Work out the finished part from the listing and answer in its coordinate system (mm). A direction names the side the tool comes from. Coordinates: 2 decimals unless noted, no trailing zeros. Write each loop counter-clockwise with the first axis right and the second up, starting at its lowest first coordinate (ties: lowest second). Pieces come first, ordered by that corner, then holes. Notation, with made-up numbers: (84.25, 39.25) - (139.25, 39.25) arc R17 ccw to (139.25, 62.25) - close; hole circle Ø3 at (-35, 2). An arc over 180 degrees is marked (long way). Answer as a JSON object with one key per item and string values. Group by question number.
from build123d import *

# Parameters (mm, degrees)
F1_DEPTH = 7
F2_R     = 5
F3_R     = 0.5
F4_R     = 1.5
F5_DEPTH = 8


with BuildPart() as f1:
    # F0 (on Top) → F1 (new body, symmetric)
    with BuildSketch(Plane.XY):
        with BuildLine():
            ThreePointArc((-5, 0), (0, -5), (5, 0))
            ThreePointArc((5, 0), (3.535534, 3.535534), (0, 5))
            ThreePointArc((0, 5), (-3.535534, 3.535534), (-5, 0))
        make_face()
        with BuildLine():
            ThreePointArc((-2.75, 2.165064), (-1.75, 3.031089), (-0.5, 3.464102))
            ThreePointArc((-0.5, 3.464102), (0, 3.5), (0.5, 3.464102))
            ThreePointArc((0.5, 3.464102), (1.75, 3.031089), (2.75, 2.165064))
            Line((2.75, 2.165064), (1.049038, 1.183013))
            Line((1.049038, 1.183013), (1.549038, 0.316987))
            Line((1.549038, 0.316987), (3.25, 1.299038))
            ThreePointArc((3.25, 1.299038), (3.5, 0), (3.25, -1.299038))
            ThreePointArc((3.25, -1.299038), (3.031089, -1.75), (2.75, -2.165064))
            ThreePointArc((2.75, -2.165064), (1.75, -3.031089), (0.5, -3.464102))
            ThreePointArc((0.5, -3.464102), (0, -3.5), (-0.5, -3.464102))
            ThreePointArc((-0.5, -3.464102), (-1.75, -3.031089), (-2.75, -2.165064))
            ThreePointArc((-2.75, -2.165064), (-3.031089, -1.75), (-3.25, -1.299038))
            ThreePointArc((-3.25, -1.299038), (-3.5, 0), (-3.25, 1.299038))
            ThreePointArc((-3.25, 1.299038), (-3.031089, 1.75), (-2.75, 2.165064))
        make_face(mode=Mode.SUBTRACT)
        with BuildLine():
            Line((-1.049038, 1.183013), (-2.75, 2.165064))
            ThreePointArc((-2.75, 2.165064), (-3.031089, 1.75), (-3.25, 1.299038))
            Line((-3.25, 1.299038), (-1.549038, 0.316987))
            Line((-1.549038, 0.316987), (-1.049038, 1.183013))
        make_face()
        with BuildLine():
            ThreePointArc((0.5, 3.464102), (0, 3.5), (-0.5, 3.464102))
            Line((-0.5, 3.464102), (-0.5, 1.5))
            Line((-0.5, 1.5), (0.5, 1.5))
            Line((0.5, 1.5), (0.5, 3.464102))
        make_face()
        with BuildLine():
            Line((-1.549038, -0.316987), (-3.25, -1.299038))
            ThreePointArc((-3.25, -1.299038), (-3.031089, -1.75), (-2.75, -2.165064))
            Line((-2.75, -2.165064), (-1.049038, -1.183013))
            Line((-1.049038, -1.183013), (-1.549038, -0.316987))
        make_face()
        with BuildLine():
            Line((-0.5, -1.5), (-0.5, -3.464102))
            ThreePointArc((-0.5, -3.464102), (0, -3.5), (0.5, -3.464102))
            Line((0.5, -3.464102), (0.5, -1.5))
            Line((0.5, -1.5), (-0.5, -1.5))
        make_face()
        with BuildLine():
            ThreePointArc((2.75, -2.165064), (3.031089, -1.75), (3.25, -1.299038))
            Line((3.25, -1.299038), (1.549038, -0.316987))
            Line((1.549038, -0.316987), (1.049038, -1.183013))
            Line((1.049038, -1.183013), (2.75, -2.165064))
        make_face()
        with BuildLine():
            ThreePointArc((-5, 0), (-3.535534, 3.535534), (0, 5))
            Line((0, 5), (-13, 5))
            Line((-13, 5), (-13, 0))
            Line((-13, 0), (-5, 0))
        make_face()
    extrude(amount=F1_DEPTH, both=True)

    # F2
    f2_edges = [f1.edges().sort_by_distance(p)[0] for p in [
        (-5, 0, 0),
    ]]
    fillet(f2_edges, radius=F2_R)

    # F3
    f3_edges = [f1.edges().sort_by_distance(p)[0] for p in [
        (-13, 5, 0),
        (-13, 0, 0),
    ]]
    fillet(f3_edges, radius=F3_R)

    # F4 (on face) → F5 (cut)
    with BuildSketch(Plane(origin=(-13, 0, 0), x_dir=(0, -1, 0), z_dir=(-1, 0, 0))):
        with Locations((-2.5, 4)):
            Circle(F4_R)
        with Locations((-2.5, -4)):
            Circle(F4_R)
    extrude(amount=-F5_DEPTH, mode=Mode.SUBTRACT)


solid = f1.part
Q1. Flat-ended cylindrical pins translate along their axes: pin 1 Ø1.6 at (y, z) = (2, -2.5) entering from +X; pin 2 Ø0.6 at (y, z) = (-2.5, -2) entering from -X; pin 3 Ø1.9 at (x, z) = (-10, 2) entering from -Y. Find the tip coordinate at first contact, or state that the pin passes through.
Q2. Section B-B on y = 1.75 is taken. Determine the outline of the cut face in (x, z), plus the area to 3 significant figures.
Q3. A tool of negligible diameter and unlimited length cuts with its end or side. For faces 1 (the face through (0, -1.5, 0)), 2 (the face through (-13, 3, 0)), 3 (the face through (-5, 3, 4)), from which of +Z, -Z, +X, -X, +Y, -Y can it reach the whole face along a straight path? Write none if from no direction.
Q4. For a pull along Z with two mould halves and no side action, classify faces 4 (the face through (-9, 1, 4)), 5 (the face through (-1.91, -1.68, 0.1)) as +Z half, -Z half, draft (parallel to the pull), parting line (faces both ways), or undercut.
Q5. Section C-C on x = 0.25 is taken. Determine the outline of the cut face in (y, z), plus the area to 3 significant figures.
Q6. Section D-D on x = -8.25 is taken. Determine the outline of the cut face in (y, z).
Q7. Consider L1, parallel to Z at x = -8.25, y = 2.5; L2, parallel to X at y = -2.25, z = 5.5; L3, parallel to X at y = 0.75, z = -0.25. Determine where each line is inside the solid, lowest interval first. Write a range as from..to.
Numbers:
{
 "1": {"pin 1": "stops at x = 4.85", "pin 2": "stops at x = -4.52", "pin 3": "stops at y = 0"},
 "2": {"outline": "(-13, -7) - (-2.03, -7) - (-2.03, 7) - (-13, 7) - (-13, 5.3) - (-5, 5.3) - (-5, 2.7) - (-13, 2.7) - (-13, -2.7) - (-5, -2.7) - (-5, -5.3) - (-13, -5.3) - close; (-0.5, -7) - (0.5, -7) - (0.5, 7) - (-0.5, 7) - close; (2.03, -7) - (4.68, -7) - (4.68, 7) - (2.03, 7) - close", "area": "163 mm²"},
 "3": {"face 1": "+Z, -Z", "face 2": "+Z, -Z, -X, +Y, -Y", "face 3": "-X"},
 "4": {"face 4": "undercut", "face 5": "draft"},
 "5": {"outline": "(-4.99, -7) - (-1.5, -7) - (-1.5, 7) - (-4.99, 7) - close; (1.5, -7) - (4.99, -7) - (4.99, 7) - (1.5, 7) - close", "area": "97.8 mm²"},
 "6": {"outline": "(-0.02, -7) - (5, -7) - (5, 7) - (-0.02, 7) - close; hole circle Ø3 at (2.5, -4); hole circle Ø3 at (2.5, 4)"},
 "7": {"L1": "z = -7..-5.5, -2.5..2.5, 5.5..7", "L2": "x = -4.48..-2.68, -0.5..0.5, 2.68..4.47", "L3": "x = -13..-3.42, -2.3..-1.3, 1.3..2.3, 3.42..4.94"}
}
